Part print with two shaded views. Sizes in mm from the minimum x, y, z corner. Round coordinates to 2 decimals unless told otherwise and drop trailing zeros. Order: outer loops, then holes, each group sorted by start corner. A loop starts at its lowest first (then second) coordinate and runs counter-clockwise, first axis right, second up. Notation, with made-up numbers: M 0.25,-33 L 13.25,-33 A25 cw 13.25,3 Z; hole C -23,-37 d7. An arc over 180 degrees is marked long. Return JSON: item names as keys, results as strings. Group by question number.
Item 1: Slice it at C-C on x = 19.05. Write the cut outline in (y, z), then the cut area to 3 significant figures.
Item 2: Probe line 1 along Y through (x, z) = (19.05, 118); line 2 along X through (y, z) = (13, 108.5). List the from-to ranges inside material, lowest first.
Item 3: Pin check, flat tips, straight feed: pin 1 Ø6 at (y, z) = (6.5, 45.5) entering from -X; pin 2 Ø3 at (x, y) = (89, 11.5) entering from +Z; pin 3 Ø5.5 at (x, y) = (88.9, 12.7) entering from -Z. Stop position of each tip, or through.
Item 4: Slice it at D-D on x = 88.9. Write the cut outline in (y, z) (3 decimals), then the cut area to 3 significant figures.
Item 5: Slice it at A-A on z = 107. Give the number of separate pieces and of enclosed holes in the cut face, then the cut area to 3 significant figures.
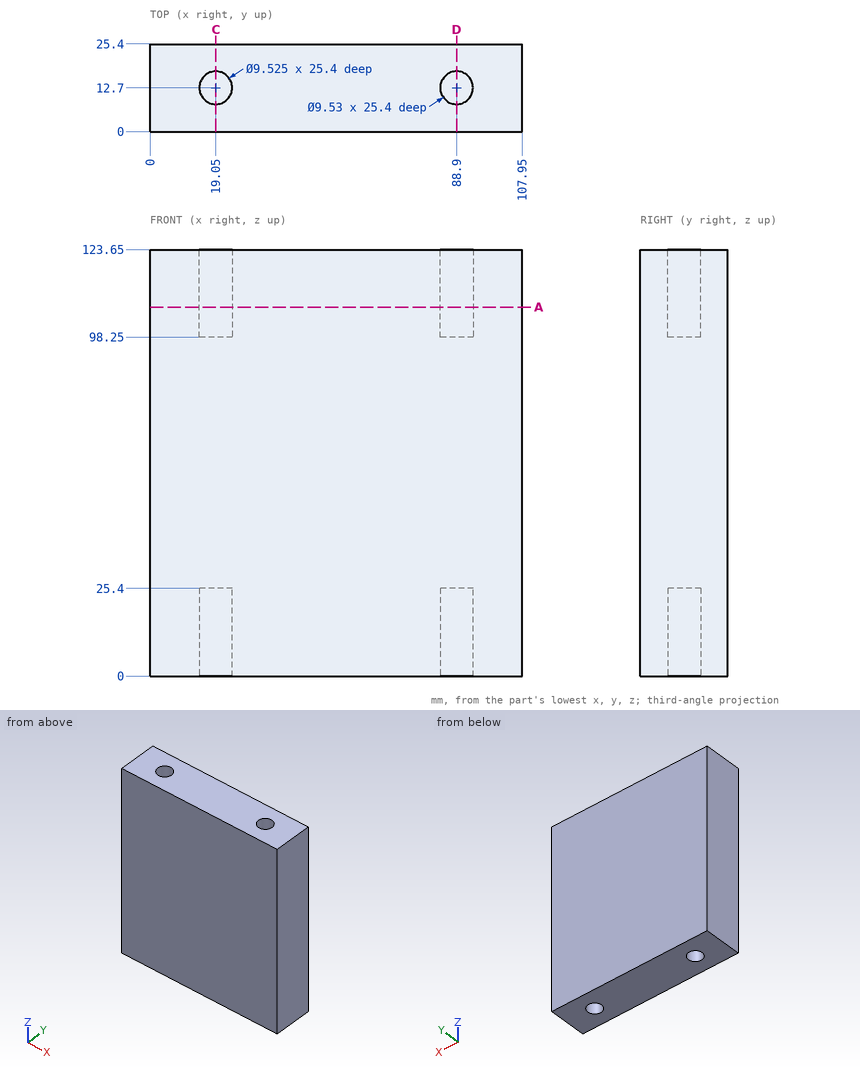
Output values:
{
 "1": {"outline": "M 0,0 L 7.94,0 L 7.94,25.4 L 17.46,25.4 L 17.46,0 L 25.4,0 L 25.4,123.65 L 17.46,123.65 L 17.46,98.25 L 7.94,98.25 L 7.94,123.65 L 0,123.65 Z", "area": "2,660 mm²"},
 "2": {"line 1": "0 to 7.94, 17.46 to 25.4", "line 2": "0 to 14.3, 23.8 to 84.14, 93.66 to 107.95"},
 "3": {"pin 1": "x = 0", "pin 2": "z = 98.25", "pin 3": "z = 25.4"},
 "4": {"outline": "M 0,0 L 7.935,0 L 7.935,25.4 L 17.465,25.4 L 17.465,0 L 25.4,0 L 25.4,123.65 L 17.465,123.65 L 17.465,98.25 L 7.935,98.25 L 7.935,123.65 L 0,123.65 Z", "area": "2,660 mm²"},
 "5": {"separate pieces": "1", "enclosed holes": "2", "area": "2,600 mm²"}
}
